For this review, take the finished solid that the model builds, in its own axes (mm). A direction names the side the tool comes from. Give positions to 0.01 mm unless a question says otherwise; leave off trailing zeros. Loops run counter-clockwise (first coordinate to the right, second up) from the corner with the lowest first, then second, coordinate; pieces in that order, holes last. Notation, with made-up numbers: (45, -37.75) - (83, -37.75) arc R26 cw to (83, -2.75) - close; hole circle Ø2 at (43.5, 10.25). An arc over 180 degrees is marked (long way). Use CSV: the item, a comma, the result in double quotes. Start each with the question number.
1. Take a section at A-A on x = -0.75. Give the boundary of the cut face in (y, z).
2. For pin 1 (3 mm diameter, centred on y = -10, z = -17, fed in from +X); pin 2 (2 mm diameter, centred on y = -8, z = -12.5, fed in from +X); pin 3 (6 mm diameter, centred on y = -10.5, z = -13, fed in from +X), all flat-tipped, find the tip position at first contact; note any pin that passes through.
3. Take a section at D-D on x = 8.75. Give the boundary of the cut face in (y, z).
4. For faces 1 (the flat face through (-3, -7, -24)), 2 (the cylindrical face through (6.67, -10.53, -23.49)), 3 (the flat face through (-3, -20.9, -12)), list the 3-axis set-ups (+Z, -Z, +X, -X, +Y, -Y) from which the entire face can be reached by the end or side of a thin tool; tool diameter is ignored.
5. Wall thickness on line 1 (Y direction, x = 1, z = -6.25); line 2 (X direction, y = -14.25, z = -16.5); line 3 (Z direction, x = 5.75, y = -20.25): over which ranges is each line inside the solid? List them lowest first.
6. Mouldability with a two-part tool opening along X and no side actions: class faces 4 (the cylindrical face through (-14.19, -19.345, -12.339)), 5 (the cylindrical face through (8.42, -19.46, -12.34)), 6 (the cylindrical face through (7.929, -18.964, -11.846)) as pulls with the +X half, pulls with the -X half, needs draft (parallel to the pull), parting line crosses it, or undercut.
7. Take a section at B-B on y = -16.75. Give the boundary of the cut face in (x, z).
```python
from build123d import *

# Parameters (mm, degrees)
EXTRUSION1_DEPTH        = 24
ENL_V_MAT_EXTRU_1_DEPTH = 1
EXTRUSION2_START        = -1
EXTRUSION2_DEPTH        = 1


with BuildPart() as part:
    # Esquisse1 → Extrusion1 (new body)
    with BuildSketch(Plane.XY):
        with BuildLine():
            Line((-8.829098079, -21.6), (3.180901921, -21.6))
            ThreePointArc((3.180901921, -21.6), (8.477131712, -19.406229791), (10.670901921, -14.11))
            Line((10.670901921, -14.11), (10.670901921, -14.1))
            ThreePointArc((10.670901921, -14.1), (8.47420278, -8.796699141), (3.170901921, -6.6))
            Line((3.170901921, -6.6), (-8.839098079, -6.6))
            ThreePointArc((-8.839098079, -6.6), (-14.13532787, -8.793770209), (-16.329098079, -14.09))
            Line((-16.329098079, -14.09), (-16.329098079, -14.1))
            ThreePointArc((-16.329098079, -14.1), (-14.132398938, -19.403300859), (-8.829098079, -21.6))
        make_face()
        with BuildLine():
            Line((3.170901921, -7.3), (-8.839098079, -7.3))
            ThreePointArc((-8.839098079, -7.3), (-13.640353124, -9.288744956), (-15.629098079, -14.09))
            Line((-15.629098079, -14.09), (-15.629098079, -14.1))
            ThreePointArc((-15.629098079, -14.1), (-13.637424191, -18.908326112), (-8.829098079, -20.9))
            Line((-8.829098079, -20.9), (3.180901921, -20.9))
            ThreePointArc((3.180901921, -20.9), (7.982156965, -18.911255044), (9.970901921, -14.11))
            Line((9.970901921, -14.11), (9.970901921, -14.1))
            ThreePointArc((9.970901921, -14.1), (7.979228033, -9.291673888), (3.170901921, -7.3))
        make_face(mode=Mode.SUBTRACT)
    extrude(amount=-EXTRUSION1_DEPTH)

    # Esquisse2 → Enlèv. mat.-Extru.1 (cut)
    with BuildSketch(Plane.XY):
        with BuildLine():
            Line((-8.829098079, -21.6), (3.180901921, -21.6))
            ThreePointArc((3.180901921, -21.6), (8.477131712, -19.406229791), (10.670901921, -14.11))
            Line((10.670901921, -14.11), (10.670901921, -14.1))
            ThreePointArc((10.670901921, -14.1), (8.47420278, -8.796699141), (3.170901921, -6.6))
            Line((3.170901921, -6.6), (-8.839098079, -6.6))
            ThreePointArc((-8.839098079, -6.6), (-14.13532787, -8.793770209), (-16.329098079, -14.09))
            Line((-16.329098079, -14.09), (-16.329098079, -14.1))
            ThreePointArc((-16.329098079, -14.1), (-14.132398938, -19.403300859), (-8.829098079, -21.6))
        make_face()
    extrude(amount=-ENL_V_MAT_EXTRU_1_DEPTH, mode=Mode.SUBTRACT)

    # Esquisse3 → Extrusion2 (add)
    with BuildSketch(Plane(origin=(0, 0, -24), x_dir=(-1, 0, 0), z_dir=(0, 0, -1)).offset(EXTRUSION2_START)):
        with BuildLine():
            Line((16.329098079, -14.1), (16.329098079, -14.09))
            ThreePointArc((16.329098079, -14.09), (14.13532787, -8.793770209), (8.839098079, -6.6))
            Line((8.839098079, -6.6), (-3.170901921, -6.6))
            ThreePointArc((-3.170901921, -6.6), (-8.47420278, -8.796699141), (-10.670901921, -14.1))
            Line((-10.670901921, -14.1), (-10.670901921, -14.11))
            ThreePointArc((-10.670901921, -14.11), (-8.477131712, -19.406229791), (-3.180901921, -21.6))
            Line((-3.180901921, -21.6), (8.829098079, -21.6))
            ThreePointArc((8.829098079, -21.6), (14.132398938, -19.403300859), (16.329098079, -14.1))
        make_face()
        with BuildLine():
            Line((8.839098079, -9.1), (-3.170901921, -9.1))
            ThreePointArc((-3.170901921, -9.1), (-6.706435827, -10.564466094), (-8.170901921, -14.1))
            Line((-8.170901921, -14.1), (-8.170901921, -14.11))
            ThreePointArc((-8.170901921, -14.11), (-6.709364759, -17.638462838), (-3.180901921, -19.1))
            Line((-3.180901921, -19.1), (8.829098079, -19.1))
            ThreePointArc((8.829098079, -19.1), (12.364631985, -17.635533906), (13.829098079, -14.1))
            Line((13.829098079, -14.1), (13.829098079, -14.09))
            ThreePointArc((13.829098079, -14.09), (12.367560918, -10.561537162), (8.839098079, -9.1))
        make_face(mode=Mode.SUBTRACT)
    extrude(amount=EXTRUSION2_DEPTH)


solid = part.part
```
Check result:
1,outline,"(-21.6, -24) - (-19.1, -24) - (-19.1, -23) - (-20.9, -23) - (-20.9, -1) - (-21.6, -1) - close; (-9.1, -24) - (-6.6, -24) - (-6.6, -1) - (-7.3, -1) - (-7.3, -23) - (-9.1, -23) - close"
2,pin 1,"stops at x = 10.21"
2,pin 2,"stops at x = 8.67"
2,pin 3,"stops at x = 10.65"
3,outline,"(-19.12, -24) - (-9.09, -24) - (-9.09, -1) - (-10.21, -1) - (-10.21, -23) - (-17.99, -23) - (-17.99, -1) - (-19.12, -1) - close"
4,face 1,"-Z, +X, -X, +Y, -Y"
4,face 2,"+Z, -Z"
4,face 3,"+Z"
5,line 1,"y = -21.6 to -20.9, -7.3 to -6.6"
5,line 2,"x = -16.33 to -15.63, 9.97 to 10.67"
5,line 3,"z = -24 to -23"
6,face 4,"pulls with the -X half"
6,face 5,"pulls with the +X half"
6,face 6,"undercut"
7,outline,"(-15.85, -24) - (-13.07, -24) - (-13.07, -23) - (-15.09, -23) - (-15.09, -1) - (-15.85, -1) - close; (7.42, -24) - (10.19, -24) - (10.19, -1) - (9.44, -1) - (9.44, -23) - (7.42, -23) - close"
